from build123d import *

# Parameters (mm, degrees)
F0_W        = 136
F0_H        = 116
F1_DEPTH    = 1
F2_W        = 11
F2_H        = 31
F2_W_2      = 16
F2_H_2      = 10
F2_W_3      = 5
F2_H_3      = 86
F2_W_4      = 10
F2_H_4      = 8
F3_DEPTH    = 10
F3_FACE_W   = 5
F3_FACE_H   = 86
F4_DEPTH    = 7.3
F3_FACE_W_2 = 16
F3_FACE_H_2 = 10
F5_DEPTH    = 8.5


with BuildPart() as f1:
    # F0 (on Top) → F1 (new body, symmetric)
    with BuildSketch(Plane.XY):
        Rectangle(F0_W, F0_H)
    extrude(amount=F1_DEPTH, both=True)

    # F2 (on face) → F3 (join)
    with BuildSketch(Plane.XY.offset(1)):
        with Locations((47.5, 17.5)):
            Rectangle(F2_W, F2_H)
        with Locations((21, 42)):
            Rectangle(F2_W_2, F2_H_2)
        with Locations((-34, 42)):
            Rectangle(F2_W_2, F2_H_2)
        with Locations((-62.5, -1)):
            Rectangle(F2_W_3, F2_H_3)
        with Locations((-49, 42)):
            Rectangle(F2_W_4, F2_H_4)
        with Locations((-19, 42)):
            Rectangle(F2_W_4, F2_H_4)
        with Locations((6, 42)):
            Rectangle(F2_W_4, F2_H_4)
        with Locations((36, 42)):
            Rectangle(F2_W_4, F2_H_4)
        with Locations((61, 30)):
            Rectangle(F2_W_4, F2_H_4)
        with Locations((61, 19.5)):
            Rectangle(F2_W_4, F2_H_4)
        with Locations((61, 9)):
            Rectangle(F2_W_4, F2_H_4)
        with Locations((61, -1.5)):
            Rectangle(F2_W_4, F2_H_4)
    extrude(amount=F3_DEPTH)

    # F3_face (on face) → F4 (cut)
    with BuildSketch(Plane(origin=(-62.5, -1, 11), x_dir=(1, 0, 0), z_dir=(0, 0, 1))):
        Rectangle(F3_FACE_W, F3_FACE_H)
    extrude(amount=-F4_DEPTH, mode=Mode.SUBTRACT)

    # F3_face (on face) → F5 (cut)
    with BuildSketch(Plane(origin=(-62.5, -1, 11), x_dir=(1, 0, 0), z_dir=(0, 0, 1))):
        with Locations((28.5, 43)):
            Rectangle(F3_FACE_W_2, F3_FACE_H_2)
        with Locations((83.5, 43)):
            Rectangle(F3_FACE_W_2, F3_FACE_H_2)
    extrude(amount=-F5_DEPTH, mode=Mode.SUBTRACT)


solid = f1.part
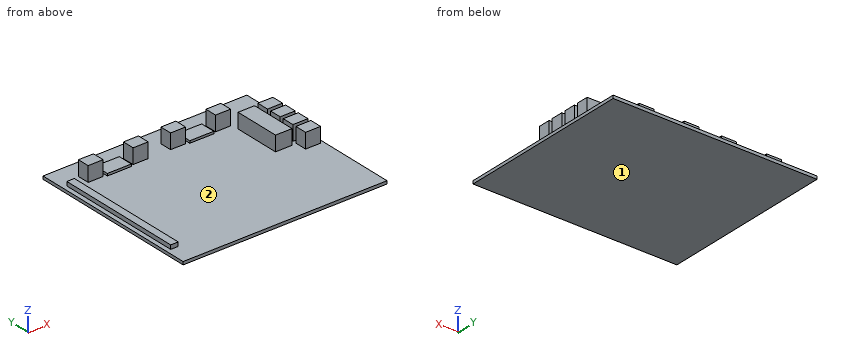
CAD build for the part. Positions are in the model's coordinates, mm. Face numbers are marked on the shaded views. Coordinates: 2 decimals unless noted, no trailing zeros. Loops run counter-clockwise (first coordinate to the right, second up) from the corner with the lowest first, then second, coordinate; pieces in that order, holes last. Notation, with made-up numbers: (23.5, 78.5) - (45.5, 78.5) arc R23 ccw to (45.5, 89.5) - close; hole circle Ø7 at (-35, -13.5). An arc over 180 degrees is marked (long way). Write item = value, one per line. Start each with the question number.
Q1. Drill centre lines: L1, parallel to Y at x = 61, z = 8.5; L2, parallel to X at y = 45.5, z = 6; L3, parallel to X at y = 8, z = 3.5. Where is each one in solid material? Low to high.
Q2. Cut at D-D, the plane y = -1. List the corners of the cut face in (x, z).
Q3. Pull direction X, two halves, no side cores. Call the marked faces 1 and 2: pulls with the +X half, pulls with the -X half, needs draft (parallel to the pull), parting line crosses it, or undercut.
Q4. Cut at B-B, the plane z = 5.25. Give the number of separate pieces and of enclosed holes in the cut face, then the cut area to 3 significant figures.
Q5. Cut at A-A, the plane y = -38. List the corners of the cut face in (x, z).
Q6. Cut at C-C, the plane x = 5. List the corners of the cut face in (y, z).
Q7. Flat gauge pins, fed straight in: pin 1 Ø2 at (x, y) = (-34.5, -32.5) entering from +Z; pin 2 Ø4 at (x, y) = (-61.5, 7) entering from +Z; pin 3 Ø5 at (x, z) = (-46.5, 4.5) entering from -Y. Where does each tip first touch, or does it go through?
Computed:
q1.L1 = -5.5 to 2.5, 5 to 13, 15.5 to 23.5, 26 to 34
q1.L2 = -54 to -44, -24 to -14, 1 to 11, 31 to 41
q1.L3 = -65 to -60, 42 to 53, 56 to 66
q2.outline = (-68, -1) - (68, -1) - (68, 1) - (66, 1) - (66, 11) - (56, 11) - (56, 1) - (-60, 1) - (-60, 3.7) - (-65, 3.7) - (-65, 1) - (-68, 1) - close
q3.face_1 = needs draft
q3.face_2 = undercut
q4.separate_pieces = 9
q4.enclosed_holes = 0
q4.area = 981 mm²
q5.outline = (-68, -1) - (68, -1) - (68, 1) - (-60, 1) - (-60, 3.7) - (-65, 3.7) - (-65, 1) - (-68, 1) - close
q6.outline = (-58, -1) - (58, -1) - (58, 1) - (46, 1) - (46, 11) - (38, 11) - (38, 1) - (-58, 1) - close
q7.pin_1 = 1
q7.pin_2 = 3.7
q7.pin_3 = 38
